Source: CAD feature listing. Evaluate the final solid. Frame: model axes, mm. A direction names the side the tool comes from. Round coordinates to 2 decimals unless told otherwise and drop trailing zeros. Loops run counter-clockwise (first coordinate to the right, second up) from the corner with the lowest first, then second, coordinate; pieces in that order, holes last. Notation, with made-up numbers: (51, 69) -> (103, 69) arc R28 ccw to (103, 91) -> close; hole circle Ø10 at (73.5, 84). An arc over 180 degrees is marked (long way). Return JSON: item names as keys, results as strings. Group by question number.
Solid Edge part; units mm, degrees
sketch "Sketch1" plane through (0, 0, 0) normal (0, -1, 0) x (1, 0, 0)
  line L0 (5, 6.3) -> (2.25, 6.3)
  line L1 (2.25, 6.3) -> (2.25, 1.5)
  line L2 (5, 1.5) -> (2.25, 1.5)
  line L3 (5, 0) -> (5, 1.5)
  line L4 (0, 0) -> (5, 0)
  line L5 (0, 7.8) -> (0, 0)
  line L6 (5, 7.8) -> (0, 7.8)
  line L7 (5, 7.8) -> (5, 6.3)
revolve "RevolvedProtrusion1" add sketch "Sketch1" angle 360 about axis through (0, 0, 7.8) along (0, 0, -1)
sketch "Sketch2" plane through (0, 0, 7.8) normal (0, 0, 1) x (1, 0, 0)
  line L0 (-1.0957, 1.2) -> (1.0957, 1.2)
  arc A0 (1.0957, 1.2) -> (-1.0957, 1.2) centre (0, 0) cw
extrude "Cutout1" cut sketch "Sketch2" against normal through all
sketch "Sketch3" plane through (0, 0, 7.8) normal (0, 0, 1) x (-1, 0, 0)
  circle A0 centre (-1.5, -3.1) radius 0.75
  circle A1 centre (1.5, -3.1) radius 0.75
extrude "Cutout2" cut sketch "Sketch3" against normal up to surface (1.5 mm away)
chamfer "Chaflán_1" distance 0.25 angle 45 4 edges at (-5, 0, 0) (-5, 0, 1.5) (-5, 0, 6.3) (-5, 0, 7.8)
sketch "Sketch4" plane through (0, 0, 0) normal (1, 0, 0) x (0, 1, 0)
  circle A0 centre (3.1, 7.8) radius 0.75
extrude "VaciadoExtruido_3" cut sketch "Sketch4" along normal mid plane 3
fillet "Redondeo_2" radius 0.5 2 edges at (-0.75, 3.1, 7.05) (0.75, 3.1, 7.05)
fillet "Redondeo_3" radius 0.25 2 edges at (2.25, 3.1, 6.3) (-0.75, 3.1, 6.3)
fillet "Redondeo_4" radius 2.5 1 edges at (-2.25, 0, 1.5)
(1) Ray query, line 1 (X direction, y = 3.1, z = 7.5); line 2 (X direction, y = -1, z = 7); line 3 (Z direction, x = 4.5, y = -2). Return the intervals inside material, ascending.
(2) Set-up query: faces 1 (the face through (-0.02, 3.12, 7.05)), 2 (the face through (0, 1.2, 4)), 3 (the face through (0, 2, 0)), 4 (the face through (-0.29, -2.23, 5.13)). Return all of +Z, -Z, +X, -X, +Y, -Y with unobstructed straight access to the full face (end or side cutting, diameter ignored); none if empty.
(3) Pin query (flat end, axial travel): pin 1 (3 mm diameter, centred on x = -1, z = 4, fed in from +Y); pin 2 (1.1 mm diameter, centred on x = -0.5, z = 2, fed in from -Y); pin 3 (3 mm diameter, centred on y = 2.5, z = 4.5, fed in from -X). Return the tip coordinate at first contact, or that it passes through.
(4) Cut plane D-D (z = 1.75). Return loops of the section in (x, y) (3 decimals).
(5) Cut plane C-C (z = 4.75). Return loops of the section in (x, y) (3 decimals).
(6) Mould query, pull axis X, two halves, no side actions, for faces 5 (the face through (-1.08, 4.88, 7.04)), 6 (the face through (2.25, 3.07, 7.18)), 7 (the face through (2, 0, 7.8)), 8 (the face through (-2.215, 2.875, 7.182)). Classes: released by +X, released by -X, zero draft, split by the parting line, or undercut.
Answers follow:
{
 "1": {"line 1": "-3.92 to -2.25, 2.25 to 3.92", "line 2": "-4.9 to -1.28, 1.28 to 4.9", "line 3": "0.17 to 1.33, 6.47 to 7.63"},
 "2": {"face 1": "+Z", "face 2": "+Z, -Z", "face 3": "-Z, +X, -X, +Y, -Y", "face 4": "none"},
 "3": {"pin 1": "y = 2.64", "pin 2": "y = -4.78", "pin 3": "x = -2.02"},
 "4": {"outline": "circle Ø7.32 at (0, 0); hole (-1.096, 1.2) arc R1.625 ccw (long way) to (1.096, 1.2) -> close"},
 "5": {"outline": "circle Ø4.5 at (0, 0); hole (-1.096, 1.2) arc R1.625 ccw (long way) to (1.096, 1.2) -> close"},
 "6": {"face 5": "split by the parting line", "face 6": "undercut", "face 7": "zero draft", "face 8": "undercut"}
}
